from build123d import *

# Parameters (mm, degrees)
ESQUISSE1_W             = 8
ESQUISSE1_H             = 36
BOSS_EXTRU_3_DEPTH      = 36
ESQUISSE9_R             = 8.1
ENL_V_MAT_EXTRU_1_DEPTH = 10
BOSS_EXTRU_4_START      = -3
ESQUISSE10_R            = 8.1
ESQUISSE10_R_2          = 4
BOSS_EXTRU_4_DEPTH      = 3
ESQUISSE13_R            = 2
ENL_V_MAT_EXTRU_2_DEPTH = 15


with BuildPart() as part:
    # Esquisse1 → Boss.-Extru.3 (new body)
    with BuildSketch(Plane(origin=(0, 0, 0), x_dir=(1, 0, 0), z_dir=(0, 1, 0))):
        with Locations((4, 18)):
            Rectangle(ESQUISSE1_W, ESQUISSE1_H)
    extrude(amount=BOSS_EXTRU_3_DEPTH)

    # Esquisse9 → Enl_v. mat.-Extru.1 (cut)
    with BuildSketch(Plane(origin=(8, 0, 0), x_dir=(0, 0, -1), z_dir=(1, 0, 0))):
        with Locations((18, 18)):
            Circle(ESQUISSE9_R)
    extrude(amount=-ENL_V_MAT_EXTRU_1_DEPTH, mode=Mode.SUBTRACT)

    # Esquisse10 → Boss.-Extru.4 (add)
    with BuildSketch(Plane.ZY.offset(BOSS_EXTRU_4_START)):
        with Locations(Location((-18, 18, 0), (0, 0, 180))):
            Circle(ESQUISSE10_R)
        with Locations((-18, 18)):
            Circle(ESQUISSE10_R_2, mode=Mode.SUBTRACT)
    extrude(amount=BOSS_EXTRU_4_DEPTH)

    # Esquisse13 → Enl_v. mat.-Extru.2 (cut)
    with BuildSketch(Plane.XZ):
        with Locations(Location((4, -4, 0), (0, 0, 270))):
            Circle(ESQUISSE13_R)
        with Locations(Location((4, -32, 0), (0, 0, 270))):
            Circle(ESQUISSE13_R)
    extrude(amount=-ENL_V_MAT_EXTRU_2_DEPTH, mode=Mode.SUBTRACT)


solid = part.part
Verification items for the finished model (mm, model axes). A direction names the side the tool comes from. Give positions to 0.01 mm unless a question says otherwise; leave off trailing zeros. Write each loop counter-clockwise with the first axis right and the second up, starting at its lowest first coordinate (ties: lowest second). Pieces come first, ordered by that corner, then holes.
(1) Cross-section at C-C (y = 7.5). Enter the section's corners in (x, z).
(2) Gauge pin test, flat ends, axial feed: pin 1 (2.5 mm diameter, centred on x = 4, z = -4, fed in from -Y); pin 2 (5 mm diameter, centred on y = 14.5, z = -21, fed in from +X). Record the tip position at first contact, or that the pin passes through.
(3) Cross-section at D-D (x = 7). Enter the section's corners in (y, z), plus the area to 3 significant figures.
(4) Mould release check, pull along Y, two halves, no side actions. Record for faces 1 (the face through (4, 0, -18)), 2 (the face through (5.54, 18.36, -9.91)), 3 (the face through (4, 18, 0)): +Y half, -Y half, draft (parallel to the pull), parting line (faces both ways), or undercut.
(5) Material ranges on line 1 (Z direction, x = 4.6, y = 18); line 2 (Z direction, x = 5.75, y = 12.5); line 3 (Y direction, x = 0.6, z = -18), recorded low to high.
(6) Cross-section at B-B (y = 18). Enter the section's corners in (x, z), plus the area to 3 significant figures.
(7) Access from +Z, -Z, +X, -X, +Y, -Y to the whole of each face (thin tool, end or side, straight path). Record for faces 4 (the face through (0, 17.7, -13.7)), 5 (the face through (4, 15, -4)), 6 (the face through (3, 20, -14)).
(8) Cross-section at A-A (z = -18). Enter the section's corners in (x, y).
Worked out:
1. outline: (0, -36) - (8, -36) - (8, 0) - (0, 0) - close; hole circle Ø4 at (4, -32); hole circle Ø4 at (4, -4)
2. pin 1: stops at y = 15
2. pin 2: stops at x = 3
3. outline: (0, -36) - (36, -36) - (36, 0) - (0, 0) - close; hole circle Ø16.2 at (18, -18)
3. area: 1,090 mm2
4. face 1: -Y half
4. face 2: undercut
4. face 3: draft
5. line 1: z = -36 to -26.1, -9.9 to 0
5. line 2: z = -36 to -32.97, -31.03 to -23.95, -12.05 to -4.97, -3.03 to 0
5. line 3: y = 0 to 14, 22 to 36
6. outline: (0, -36) - (8, -36) - (8, -26.1) - (3, -26.1) - (3, -22) - (0, -22) - close; (0, -14) - (3, -14) - (3, -9.9) - (8, -9.9) - (8, 0) - (0, 0) - close
6. area: 183 mm2
7. face 4: +Z, -Z, -X, +Y, -Y
7. face 5: -Y
7. face 6: +X
8. outline: (0, 0) - (8, 0) - (8, 9.9) - (3, 9.9) - (3, 14) - (0, 14) - close; (0, 22) - (3, 22) - (3, 26.1) - (8, 26.1) - (8, 36) - (0, 36) - close
